Check sheet for the modelled part. Datum: model origin and axes. Units: mm. Face numbers are marked on the shaded views. A direction names the side the tool comes from. Give positions to 0.01 mm unless a question says otherwise; leave off trailing zeros. Loops run counter-clockwise (first coordinate to the right, second up) from the corner with the lowest first, then second, coordinate; pieces in that order, holes last. Notation, with made-up numbers: M -7.5,-35 L 26.5,-35 A12 ccw 26.5,-25 Z; hole C 5.5,29.25 d11. An arc over 180 degrees is marked long. Use one line per item in the form item = value.
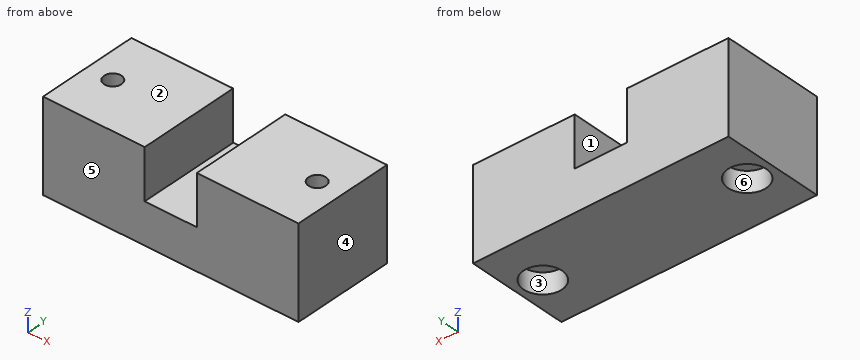
from build123d import *

# Parameters (mm, degrees)
SKETCH2_W           = 50
SKETCH2_H           = 20
SKETCH2_R           = 1.7
BOSS_EXTRUDE1_DEPTH = 8
BOSS_EXTRUDE2_DEPTH = 20
SKETCH6_R           = 3.75
CUT_EXTRUDE1_DEPTH  = 4
SKETCH7_R           = 1.7
CUT_EXTRUDE2_DEPTH  = 18.8


with BuildPart() as part:
    # Sketch2 → Boss-Extrude1 (new body)
    with BuildSketch(Plane.XY):
        Rectangle(SKETCH2_W, SKETCH2_H)
        with Locations((-20, 0)):
            Circle(SKETCH2_R, mode=Mode.SUBTRACT)
        with Locations((20, 0)):
            Circle(SKETCH2_R, mode=Mode.SUBTRACT)
    extrude(amount=BOSS_EXTRUDE1_DEPTH)

    # Sketch5 → Boss-Extrude2 (add)
    with BuildSketch(Plane.XZ.offset(10)):
        with BuildLine():
            Line((-25, 8), (-25, 17.8))
            Line((-25, 17.8), (-5.1, 17.8))
            Line((-5.1, 17.8), (-5.1, 8))
            Line((-5.1, 8), (5.1, 8))
            Line((5.1, 8), (5.1, 17.8))
            Line((5.1, 17.8), (25, 17.8))
            Line((25, 17.8), (25, 8))
            ThreePointArc((25, 8), (0, 0), (-25, 8))
        make_face()
    extrude(amount=-BOSS_EXTRUDE2_DEPTH)

    # Sketch6 → Cut-Extrude1 (cut)
    with BuildSketch(Plane(origin=(0, 0, 0), x_dir=(-1, 0, 0), z_dir=(0, 0, -1))):
        with Locations((20, 0)):
            Circle(SKETCH6_R)
        with Locations((-20, 0)):
            Circle(SKETCH6_R)
    extrude(amount=-CUT_EXTRUDE1_DEPTH, mode=Mode.SUBTRACT)

    # Sketch7 → Cut-Extrude2 (cut, through all)
    with BuildSketch(Plane(origin=(0, 0, 0), x_dir=(-1, 0, 0), z_dir=(0, 0, -1))):
        with Locations((20, 0)):
            Circle(SKETCH7_R)
        with Locations((-20, 0)):
            Circle(SKETCH7_R)
    extrude(amount=-CUT_EXTRUDE2_DEPTH, mode=Mode.SUBTRACT)


solid = part.part
1) Section check A-A (z = 11.5). Record the cut outline in (x, y).
Evaluation:
outline = M -25,-10 L -5.1,-10 L -5.1,10 L -25,10 Z; M 5.1,-10 L 25,-10 L 25,10 L 5.1,10 Z; hole C -20,0 d3.4; hole C 20,0 d3.4
2) Release check for a two-part mould opening along Y. For the marked faces 4, 5 and 6 record: pulls with the +Y half, pulls with the -Y half, needs draft (parallel to the pull), parting line crosses it, or undercut.
Evaluation:
face_4 = needs draft
face_5 = pulls with the -Y half
face_6 = undercut
3) Scan lines: line 1 (X direction, y = 0, z = 9.75); line 2 (X direction, y = 0, z = 5); line 3 (Y direction, x = -20, z = 1.85). Record each from-to range of solid material in increasing order.
Evaluation:
line_1 = -25 to -21.7, -18.3 to -5.1, 5.1 to 18.3, 21.7 to 25
line_2 = -25 to -21.7, -18.3 to 18.3, 21.7 to 25
line_3 = -10 to -3.75, 3.75 to 10
4) Set-up check for the marked faces 1, 2 and 3: record each of +Z, -Z, +X, -X, +Y, -Y from which the full face is reachable in a straight line by a thin tool's end or side.
Evaluation:
face_1 = +Z, +Y, -Y
face_2 = +Z, +X, -X, +Y, -Y
face_3 = -Z
5) Section check D-D (y = 4.5). Record the cut outline in (x, z), then the cut area to 3 significant figures.
Evaluation:
outline = M -25,0 L 25,0 L 25,17.8 L 5.1,17.8 L 5.1,8 L -5.1,8 L -5.1,17.8 L -25,17.8 Z
area = 790 mm^2
6) Section check B-B (y = 0). Record the cut outline in (x, z).
Evaluation:
outline = M -25,0 L -23.75,0 L -23.75,4 L -21.7,4 L -21.7,17.8 L -25,17.8 Z; M -18.3,4 L -16.25,4 L -16.25,0 L 16.25,0 L 16.25,4 L 18.3,4 L 18.3,17.8 L 5.1,17.8 L 5.1,8 L -5.1,8 L -5.1,17.8 L -18.3,17.8 Z; M 21.7,4 L 23.75,4 L 23.75,0 L 25,0 L 25,17.8 L 21.7,17.8 Z
7) Section check C-C (x = -20). Record the cut outline in (y, z).
Evaluation:
outline = M -10,0 L -3.75,0 L -3.75,4 L -1.7,4 L -1.7,17.8 L -10,17.8 Z; M 1.7,4 L 3.75,4 L 3.75,0 L 10,0 L 10,17.8 L 1.7,17.8 Z
8) Depth check by flat-ended pin: pin 1 Ø4.5 at (x, y) = (20, 0) entering from -Z; pin 2 Ø2 at (x, y) = (-20, 0) entering from -Z; pin 3 Ø2 at (x, y) = (-0.5, -2.5) entering from +Z. Enter the tip coordinate at first touch or a pass-through.
Evaluation:
pin_1 = 4
pin_2 = through
pin_3 = 8
